For this review, take the finished solid that the model builds, in its own axes (mm). A direction names the side the tool comes from. Coordinates: 2 decimals unless noted, no trailing zeros. Order: outer loops, then holes, each group sorted by start corner. A loop starts at its lowest first (then second) coordinate and runs counter-clockwise, first axis right, second up. Notation, with made-up numbers: (-40, 53) -> (10, 53) arc R27 cw to (10, 71) -> close; hole circle Ø8 at (23.25, 42.25). An arc over 180 degrees is marked (long way). Return JSON: item names as keys, results as strings. Group by question number.
Item 1: Take a section at B-B (z = 15.5). Write out the cut boundary in (x, y), then the cut area to 3 significant figures.
Item 2: For line 1 along X through (y, z) = (-23, 4.2); line 2 along Y through (x, z) = (-40.5, 5.35); line 3 along Y through (x, z) = (2, 23), list the stretches that pass through material, from the lowest coordinate up.
Item 3: Take a section at A-A (x = -40.5). Write out the cut boundary in (y, z).
Item 4: Insertion check: pin 1 (0.7 mm diameter, centred on x = 24.5, y = 15, fed in from -Z); pin 2 (4 mm diameter, centred on y = -14, z = 22.5, fed in from +X); pin 3 (8 mm diameter, centred on x = -40.5, y = 23, fed in from -Z). Each pin has a flat end and moves straight along its axis. Give the tip position at first contact, or say it passes through.
Item 5: Draft analysis for pull direction X (two halves, no side actions). For faces 4 (the cylindrical face through (-15.798, -15.128, 11.945)), 5 (the flat face through (0, 20, 6)), 6 (the cylindrical face through (-4.03, 15.13, 35.44)), state which applies: +X half, -X half, draft (parallel to the pull), parting line (faces both ways), or undercut.
Item 6: Take a section at C-C (x = -4). Write out the cut boundary in (y, z).
Item 7: Machinability: for faces 1 (the flat face through (32.471, 24.356, 4.722)), 2 (the cylindrical face through (-2.283, 15.128, 31.216)), 3 (the flat face through (-28.006, -29.758, 5.207)), which of the approach directions +Z, -Z, +X, -X, +Y, -Y give a long, thin tool a straight path to every point of the face, cutting with its end or side? Answer none if there is none.
Item 8: Take a section at D-D (y = 0). Write out the cut boundary in (x, z), then the cut area to 3 significant figures.
```python
from build123d import *

# Parameters (mm, degrees)
SKETCH_R        = 3.5
SKETCH_R_2      = 6
PAD_DEPTH       = 9
POCKET001_DEPTH = 75
POCKET_DEPTH    = 75
SKETCH003_R     = 4
PAD001_DEPTH    = 3.2


with BuildPart() as part:
    # Sketch → Pad (new body)
    with BuildSketch(Plane.XY):
        with BuildLine():
            Line((-34.169398, 37.323843), (-51.754493, 32.696186))
            ThreePointArc((-51.754493, 32.696186), (-52.291989, 32.339647), (-52.5, 31.729111))
            Line((-52.5, 31.729111), (-52.5, -31.729111))
            ThreePointArc((-52.5, -31.729111), (-52.291989, -32.339647), (-51.754493, -32.696186))
            Line((-51.754493, -32.696186), (-34.169398, -37.323843))
            ThreePointArc((-34.169398, -37.323843), (-33.573754, -37.296777), (-33.099398, -36.935515))
            Line((-33.099398, -36.935515), (-22.767161, -22.376454))
            ThreePointArc((-22.040194, -21.959128), (-22.449515, -22.087944), (-22.767161, -22.376454))
            Line((-22.040194, -21.959128), (22.160937, -18.030139))
            ThreePointArc((22.787034, -18.182984), (22.486636, -18.054741), (22.160937, -18.030139))
            Line((22.787034, -18.182984), (41.886908, -30.359154))
            ThreePointArc((41.886908, -30.359154), (42.485559, -30.514059), (43.060848, -30.2873))
            Line((43.060848, -30.2873), (52.136383, -22.799984))
            ThreePointArc((52.136383, -22.799984), (52.404539, -22.455001), (52.5, -22.028611))
            Line((52.5, -22.028611), (52.5, 22.028611))
            ThreePointArc((52.5, 22.028611), (52.404539, 22.455001), (52.136383, 22.799984))
            Line((52.136383, 22.799984), (43.060848, 30.2873))
            ThreePointArc((43.060848, 30.2873), (42.485559, 30.514059), (41.886908, 30.359154))
            Line((41.886908, 30.359154), (22.787034, 18.182984))
            ThreePointArc((22.160937, 18.030139), (22.486636, 18.054741), (22.787034, 18.182984))
            Line((22.160937, 18.030139), (-22.040194, 21.959128))
            ThreePointArc((-22.767161, 22.376454), (-22.449515, 22.087944), (-22.040194, 21.959128))
            Line((-22.767161, 22.376454), (-33.099398, 36.935515))
            ThreePointArc((-33.099398, 36.935515), (-33.573754, 37.296777), (-34.169398, 37.323843))
        make_face()
        with Locations((-40.5, 0)):
            Circle(SKETCH_R, mode=Mode.SUBTRACT)
        with Locations((-40.5, 23)):
            Circle(SKETCH_R, mode=Mode.SUBTRACT)
        with Locations((-40.5, -23)):
            Circle(SKETCH_R, mode=Mode.SUBTRACT)
        with Locations((12.5, 0)):
            Circle(SKETCH_R_2, mode=Mode.SUBTRACT)
    extrude(amount=PAD_DEPTH)

    # Sketch006 → Pocket001 (cut)
    with BuildSketch(Plane.XZ.offset(37.5)):
        with BuildLine():
            ThreePointArc((52.5, 4.5), (0, 8.9), (-52.5, 4.5))
            Line((-52.5, 4.5), (-52.5, 9))
            Line((52.5, 9), (-52.5, 9))
            Line((52.5, 4.5), (52.5, 9))
        make_face()
    extrude(amount=-POCKET001_DEPTH, mode=Mode.SUBTRACT)

    # Sketch005 → Pocket (cut)
    with BuildSketch(Plane.XZ.offset(37.5)):
        with BuildLine():
            ThreePointArc((52.516865, 0), (0.003551, 4.000338), (-52.509762, 0))
            Line((-52.509762, 0), (52.516865, 0))
        make_face()
    extrude(amount=-POCKET_DEPTH, mode=Mode.SUBTRACT)

    # Sketch003 (on DatumPlane) → Pad001 (join)
    with BuildSketch(Plane.XZ.offset(13.55)):
        with BuildLine():
            ThreePointArc((6.737796, 27.25), (-4.240883, 35.380569), (-8.816593, 22.508102))
            ThreePointArc((-27.473413, 8), (-15.656455, 12.053882), (-8.816593, 22.508102))
            Line((-27.473413, 8), (25.987796, 8))
            ThreePointArc((6.737796, 27.25), (12.37599, 13.638194), (25.987796, 8))
        make_face()
        with Locations((-1.762204, 27.25)):
            Circle(SKETCH003_R, mode=Mode.SUBTRACT)
    pad001 = extrude(amount=PAD001_DEPTH)

    # Mirrored: Pad001 across XZ
    add(pad001.mirror(Plane.XZ))


solid = part.part
```
Findings below:
{
 "1": {"outline": "(-12.23, -16.75) -> (10.74, -16.75) -> (10.74, -13.55) -> (-12.23, -13.55) -> close; (-12.23, 13.55) -> (10.74, 13.55) -> (10.74, 16.75) -> (-12.23, 16.75) -> close", "area": "147 mm2"},
 "2": {"line 1": "x = -52.5 to -44, -37 to -23.21, 30.34 to 51.89", "line 2": "y = -35.66 to -26.5, -19.5 to -3.5, 3.5 to 19.5, 26.5 to 35.66", "line 3": "y = -16.75 to -13.55, 13.55 to 16.75"},
 "3": {"outline": "(-35.66, 1.63) -> (-26.5, 1.63) -> (-26.5, 6.29) -> (-35.66, 6.29) -> close; (-19.5, 1.63) -> (-3.5, 1.63) -> (-3.5, 6.29) -> (-19.5, 6.29) -> close; (3.5, 1.63) -> (19.5, 1.63) -> (19.5, 6.29) -> (3.5, 6.29) -> close; (26.5, 1.63) -> (35.66, 1.63) -> (35.66, 6.29) -> (26.5, 6.29) -> close"},
 "4": {"pin 1": "stops at z = 3.11", "pin 2": "stops at x = 7.96", "pin 3": "stops at z = 1.13"},
 "5": {"face 4": "-X half", "face 5": "undercut", "face 6": "parting line"},
 "6": {"outline": "(-20.36, 3.98) -> (20.36, 3.98) -> (20.36, 8.87) -> (16.75, 8.87) -> (16.75, 23.93) -> (13.55, 23.93) -> (13.55, 8.87) -> (-13.55, 8.87) -> (-13.55, 23.93) -> (-16.75, 23.93) -> (-16.75, 8.87) -> (-20.36, 8.87) -> close; (-16.75, 30.57) -> (-13.55, 30.57) -> (-13.55, 35.45) -> (-16.75, 35.45) -> close; (13.55, 30.57) -> (16.75, 30.57) -> (16.75, 35.45) -> (13.55, 35.45) -> close"},
 "7": {"face 1": "+Z, -Z, +Y", "face 2": "+Y, -Y", "face 3": "+Z, -Z, -Y"},
 "8": {"outline": "(-52.5, 0) arc R346.68 cw to (-44, 1.2) -> (-44, 5.82) arc R315.41 ccw to (-52.5, 4.5) -> close; (-37, 2.02) arc R346.68 cw to (6.5, 3.94) -> (6.5, 8.83) arc R315.41 ccw to (-37, 6.72) -> close; (18.5, 3.51) arc R346.68 cw to (52.5, 0) -> (52.5, 4.5) arc R315.41 ccw to (18.5, 8.36) -> close", "area": "409 mm2"}
}
